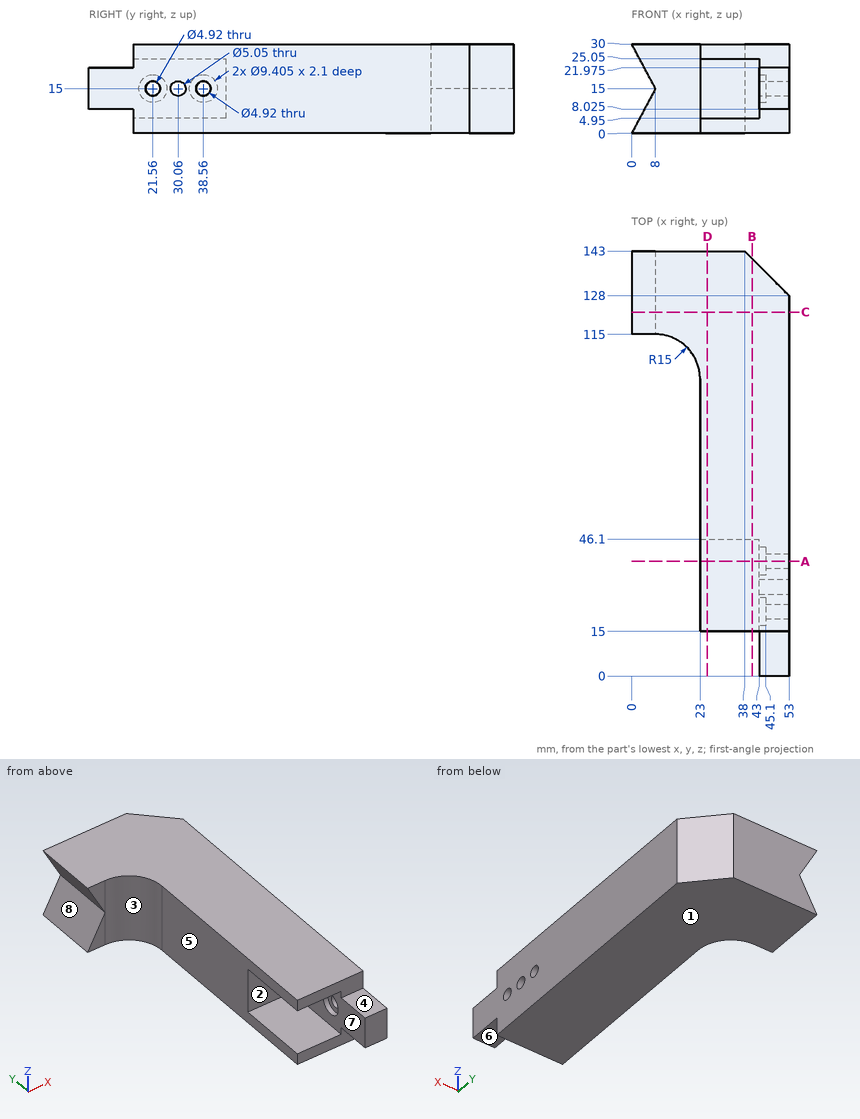
The drawing under review shows one solid part. Ordinate dimensions are in mm from its lowest x, y, z. A direction names the side the tool comes from. Coordinates: 2 decimals unless noted, no trailing zeros. Order: outer loops, then holes, each group sorted by start corner. A loop starts at its lowest first (then second) coordinate and runs counter-clockwise, first axis right, second up. Notation, with made-up numbers: (-20, 71.25) -> (28, 71.25) arc R22 cw to (28, 94.25) -> close; hole circle Ø1 at (31.25, -30.5). An arc over 180 degrees is marked (long way). One line per item, written item: value.
1) Draft analysis for pull direction Z (two halves, no side actions). For the marked faces 1, 2 and 3, state which applies: +Z half, -Z half, draft (parallel to the pull), parting line (faces both ways), or undercut.
Output values:
face 1: -Z half
face 2: undercut
face 3: draft
2) We need section B-B, the plane x = 40.5. Give the boundary of the cut face in (y, z).
Output values:
outline: (15, 0) -> (140.5, 0) -> (140.5, 30) -> (15, 30) -> (15, 25.05) -> (46.1, 25.05) -> (46.1, 4.95) -> (15, 4.95) -> close
3) We need section D-D, the plane x = 25.5. Give the boundary of the cut face in (y, z), then the cut area to 3 significant figures.
Output values:
outline: (15, 0) -> (143, 0) -> (143, 30) -> (15, 30) -> (15, 25.05) -> (46.1, 25.05) -> (46.1, 4.95) -> (15, 4.95) -> close
area: 3,210 mm2
4) Clearance check with flat-ended pins moving along their axes: P1, Ø5, axis at x = 50, y = 9, coming from the -Z side (3 decimals); P2, Ø8, axis at x = 46, y = 5, coming from the +Z side (3 decimals); P3, Ø9, axis at x = 37, z = 3.5, coming from the -Y side. State where each tip first meets the part, or that it passes through.
Output values:
P1: stops at z = 8.025
P2: stops at z = 21.975
P3: stops at y = 15
5) We need section C-C, the plane y = 122.5. Give the boundary of the cut face in (x, z), then the cut area to 3 significant figures.
Output values:
outline: (0, 0) -> (53, 0) -> (53, 30) -> (0, 30) -> (8, 15) -> close
area: 1,470 mm2
6) To check wall thickness, follow probe 1 along Y at (x, z) = (43.4, 15) (1 decimal); probe 2 along Z at (x, y) = (40, 37); probe 3 along Z at (x, y) = (46, 30). State the ranges of each line that lie inside material, in increasing order. Write a range as [from, to].
Output values:
probe 1: y = [0, 16.9], [26.3, 27.5], [32.6, 33.9], [43.3, 137.6]
probe 2: z = [0, 4.95], [25.05, 30]
probe 3: z = [0, 12.48], [17.52, 30]
7) Machinability: for the marked faces 4, 5, 6, 7 and 8, which of the approach directions +Z, -Z, +X, -X, +Y, -Y give a long, thin tool a straight path to every point of the face, cutting with its end or side? Answer none if there is none.
Output values:
face 4: +Z, +X, -X, -Y
face 5: +Z, -Z, -X, -Y
face 6: -Z, +X, -X, -Y
face 7: -X, -Y
face 8: -X, +Y, -Y
8) We need section A-A, the plane y = 38.56. Give the boundary of the cut face in (x, z).
Output values:
outline: (23, 0) -> (53, 0) -> (53, 12.54) -> (45.1, 12.54) -> (45.1, 10.3) -> (43, 10.3) -> (43, 4.95) -> (23, 4.95) -> close; (23, 25.05) -> (43, 25.05) -> (43, 19.7) -> (45.1, 19.7) -> (45.1, 17.46) -> (53, 17.46) -> (53, 30) -> (23, 30) -> close
